The figure shows three views and two pictorial views of one solid part (mm, origin at its lowest corner). Answer the questions. Coordinates: 2 decimals unless noted, no trailing zeros. Order: outer loops, then holes, each group sorted by start corner. A loop starts at its lowest first (then second) coordinate and runs counter-clockwise, first axis right, second up. Notation, with made-up numbers: (41.25, 73.5) - (70.25, 73.5) arc R5 cw to (70.25, 81.5) - close; hole circle Ø11 at (15, 61). An arc over 180 degrees is marked (long way). Use one line per item in the form item = value. Start each with the question number.
Item 1: This flat-tipped pin is pushed along its axis until it touches: pin 1 Ø2 at (x, z) = (11.5, 28) entering from -Y. Where does it stop, or does it pass through?
Item 2: Section B-B, the plane z = 62 is taken. Write down the section's boundary in (x, y) (1 decimal).
Item 3: Section C-C, the plane y = 23 is taken. Write down the section's boundary in (x, z) (1 decimal).
Item 4: Consider line 1 along Y through (x, z) = (46.5, 52.5); line 2 along Z through (x, y) = (63.5, 4); line 3 along X through (y, z) = (3, 35) (1 decimal). Determine where each line is inside the solid, lowest interval first. Write a range as [from, to].
Item 5: Section A-A, the plane x = 35.5 is taken. Write down the section's boundary in (y, z) (1 decimal).
Item 6: The mould has two halves that part along Z. Classify the marked faces 1, 2 and 3: released by +Z, released by -Z, zero draft, split by the parting line, or undercut.
Item 7: Section D-D, the plane x = 6.5 is taken. Write down the section's boundary in (y, z) (1 decimal).
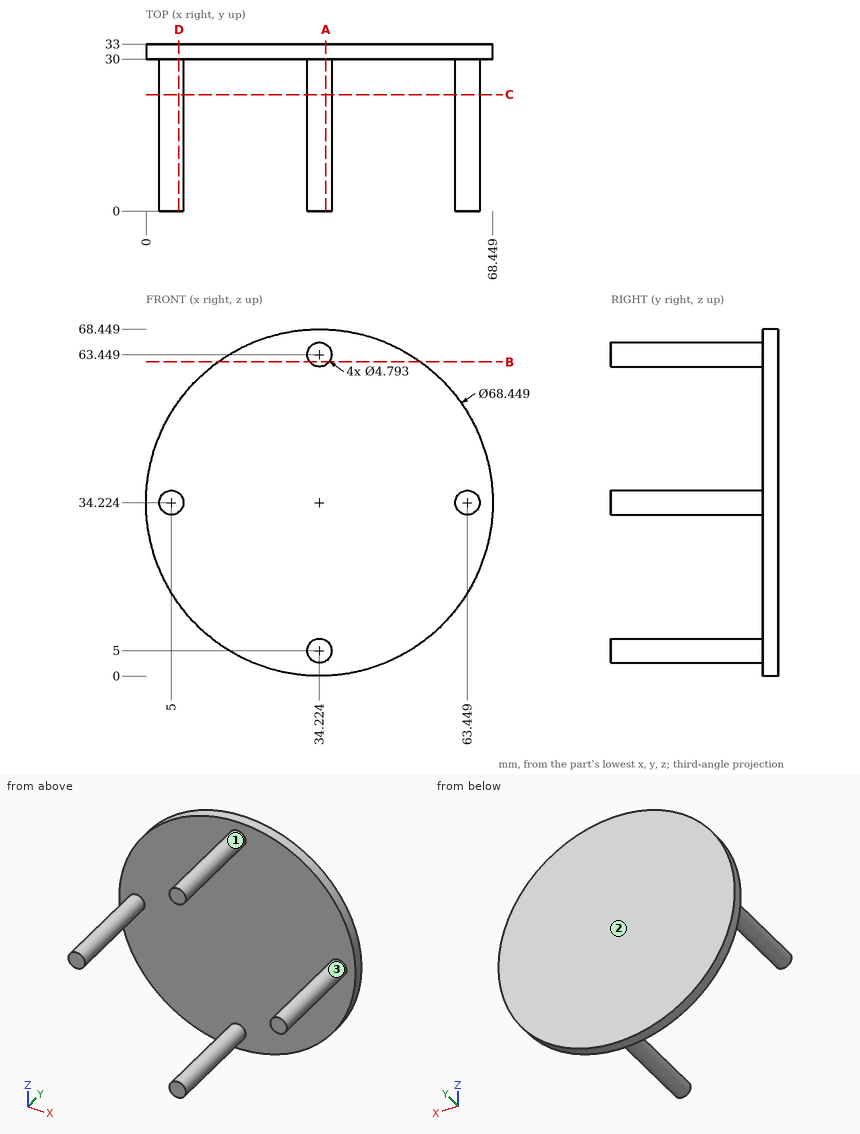
Response:
q1.pin_1 = 30
q2.outline = (14.2, 30) - (32.3, 30) - (32.3, 0) - (36.1, 0) - (36.1, 30) - (54.2, 30) - (54.2, 33) - (14.2, 33) - close
q3.outline = circle Ø4.8 at (5, 34.2); circle Ø4.8 at (34.2, 5); circle Ø4.8 at (34.2, 63.4); circle Ø4.8 at (63.4, 34.2)
q4.line_1 = [30, 33]
q4.line_2 = [31.83, 36.62]
q4.line_3 = [2.7, 7.3], [61.2, 65.7]
q5.outline = (0, 3) - (30, 3) - (30, 0) - (33, 0) - (33, 68.4) - (30, 68.4) - (30, 65.5) - (0, 65.5) - (0, 61.4) - (30, 61.4) - (30, 7) - (0, 7) - close
q6.face_1 = undercut
q6.face_2 = zero draft
q6.face_3 = split by the parting line
q7.outline = (0, 32.4) - (30, 32.4) - (30, 14.2) - (33, 14.2) - (33, 54.3) - (30, 54.3) - (30, 36.1) - (0, 36.1) - close
